Source: CAD feature listing. Evaluate the final solid. Frame: model axes, mm. Round coordinates to 2 decimals unless told otherwise and drop trailing zeros. Loops run counter-clockwise (first coordinate to the right, second up) from the corner with the lowest first, then second, coordinate; pieces in that order, holes last. Notation, with made-up numbers: M -20.5,-5 L -14.5,-5 A30 cw -14.5,18 Z; hole C 56.5,71 d5. An arc over 180 degrees is marked long. Write each question's results on one line, items separated by ' | '. Start each with the question number.
1. Section B-B on y = -1.25. Output: boundary loops of the cut face in (x, z), and give its area (3 significant figures).
2. Ray query, line 1 (Z direction, x = 0.5, y = -3); line 2 (X direction, y = -1, z = -0.65). Return the intervals inside material, ascending.
3. Section A-A on x = 0.25. Output: boundary loops of the cut face in (y, z).
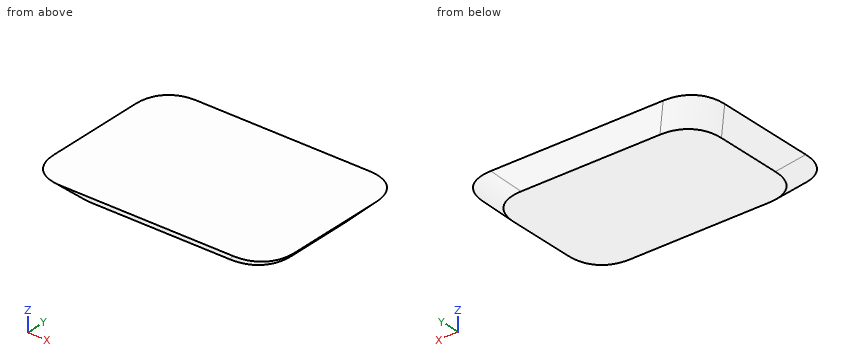
Autodesk Inventor part; units mm, degrees
ref_plane "YZ Plane" through (0, 0, 0) normal (1, 0, 0) x (0, 1, 0)
ref_plane "XZ Plane" through (0, 0, 0) normal (0, 1, 0) x (-1, 0, 0)
ref_plane "XY Plane" through (0, 0, 0) normal (0, 0, 1) x (1, 0, 0)
sketch "Sketch1" plane through (0, 0, 0) normal (0, 0, 1) x (1, 0, 0)
  line L0 (-5, -3.5) -> (5, -3.5)
  line L1 (5, -3.5) -> (5, 3.5)
  line L2 (5, 3.5) -> (-5, 3.5)
  line L3 (-5, 3.5) -> (-5, -3.5)
  line L4 (-5, -3.5) -> (5, 3.5) construction
  line L5 (5, -3.5) -> (-5, 3.5) construction
  point P0 (0, 0)
  dimension "d0" = 10
  dimension "d1" = 7
extrude "Extrusion1" add sketch "Sketch1" against normal blind 0.7 draft -45
fillet "Fillet1" radius 2 4 edges at (-4.65, -3.15, -0.35) (-4.65, 3.15, -0.35) (4.65, -3.15, -0.35) (4.65, 3.15, -0.35)
properties part number "Base"
Taken from the geometry:
1) outline: M -5,0 L -4.3,-0.7 L 4.3,-0.7 L 5,0 Z | area: 6.51 mm^2
2) line 1: -0.5 to 0 | line 2: -4.35 to 4.35
3) outline: M -3.5,0 L -2.8,-0.7 L 2.8,-0.7 L 3.5,0 Z
